Geometry check sheet. Reference: drawing and pictorial views, mm from the part's lowest x, y, z. Give positions to 0.01 mm unless a question says otherwise; leave off trailing zeros. Write each loop counter-clockwise with the first axis right and the second up, starting at its lowest first coordinate (ties: lowest second). Pieces come first, ordered by that corner, then holes. Notation, with made-up numbers: (-28.5, -0.75) -> (-23.5, -0.75) arc R14 cw to (-23.5, 3.25) -> close; hole circle Ø6 at (-32.75, -5.75). An arc over 180 degrees is marked (long way). Use a Markdown table: item, result. Add a question column.
1. Cross-section at A-A (z = 0.15). Enter the section's corners in (x, y).
2. Cross-section at B-B (y = 31). Enter the section's corners in (x, z), then the cut area to 3 significant figures.
3. Scan lines: probe 1 along Y at (x, z) = (17, 0.3); probe 2 along Y at (x, z) = (17.5, 0.5); probe 3 along Y at (x, z) = (19.25, 0.75). Record each from-to range of solid material in increasing order. Write a range as [from, to].
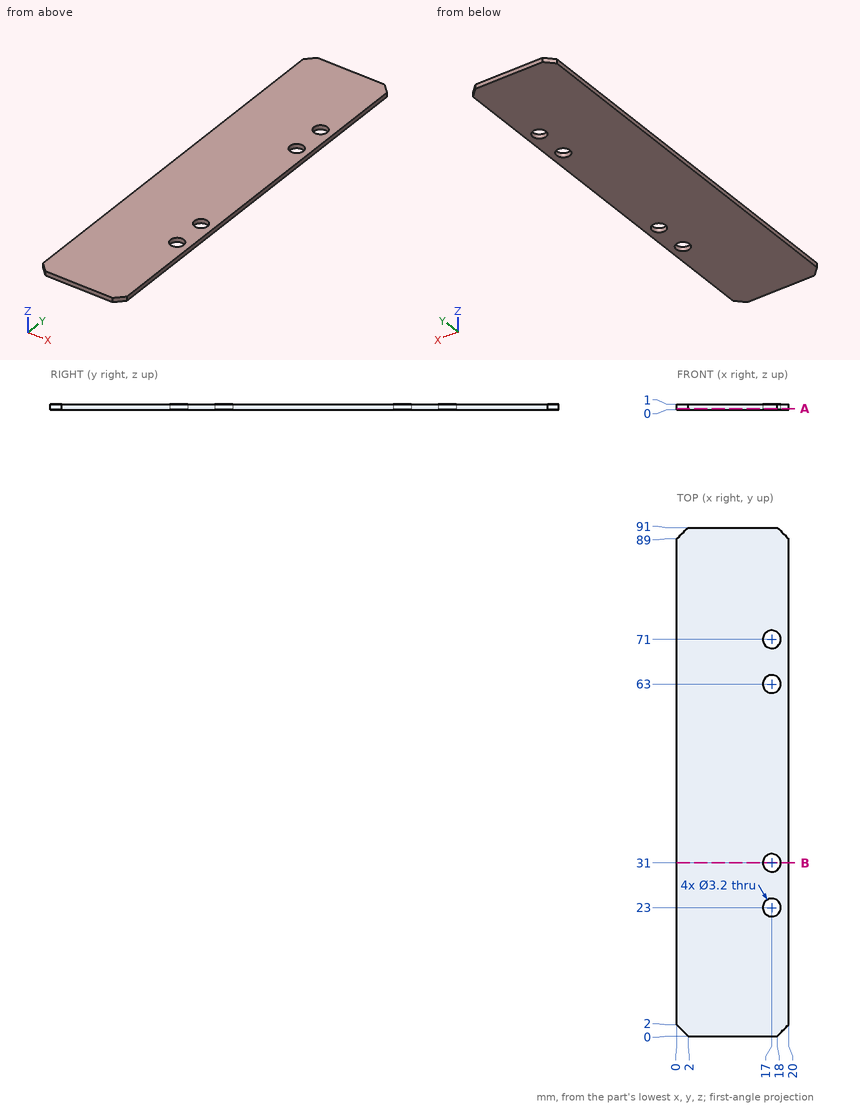
Worked answers:
| question | item | result |
|---|---|---|
| 1 | outline | (0, 2) -> (2, 0) -> (18, 0) -> (20, 2) -> (20, 89) -> (18, 91) -> (2, 91) -> (0, 89) -> close; hole circle Ø3.2 at (17, 23); hole circle Ø3.2 at (17, 31); hole circle Ø3.2 at (17, 63); hole circle Ø3.2 at (17, 71) |
| 2 | outline | (0, 0) -> (15.4, 0) -> (15.4, 1) -> (0, 1) -> close; (18.6, 0) -> (20, 0) -> (20, 1) -> (18.6, 1) -> close |
| 2 | area | 16.8 mm² |
| 3 | probe 1 | y = [0, 21.4], [24.6, 29.4], [32.6, 61.4], [64.6, 69.4], [72.6, 91] |
| 3 | probe 2 | y = [0, 21.48], [24.52, 29.48], [32.52, 61.48], [64.52, 69.48], [72.52, 91] |
| 3 | probe 3 | y = [1.25, 89.75] |
